The model under review builds one solid part; all positions refer to its coordinate system, in mm. Face numbers are marked on the shaded views. Coordinates: 2 decimals unless noted, no trailing zeros. Order: outer loops, then holes, each group sorted by start corner. A loop starts at its lowest first (then second) coordinate and runs counter-clockwise, first axis right, second up. Notation, with made-up numbers: (45, 20.5) -> (51, 20.5) arc R17 ccw to (51, 38.5) -> close; hole circle Ø8 at (-30.5, -14). An arc over 180 degrees is marked (long way). Answer as CSV lines item,"result". Start each with the question number.
from build123d import *

# Parameters (mm, degrees)
SKETCH1_R           = 52.832
SKETCH1_R_2         = 50.8
BOSS_EXTRUDE1_DEPTH = 457.2
CUT_EXTRUDE1_DEPTH  = 464.264805967
CIRPATTERN1_COUNT   = 8


with BuildPart() as part:
    # Sketch1 → Boss-Extrude1 (new body)
    with BuildSketch(Plane(origin=(0, 0, 0), x_dir=(1, 0, 0), z_dir=(0, 1, 0))):
        with Locations(Location((0, 0, 0), (0, 0, 270))):
            Circle(SKETCH1_R)
        with Locations(Location((0, 0, 0), (0, 0, 270))):
            Circle(SKETCH1_R_2, mode=Mode.SUBTRACT)
    extrude(amount=BOSS_EXTRUDE1_DEPTH)

    # Sketch2 → Cut-Extrude1 (cut, through all)
    with BuildSketch(Plane.XY):
        with BuildLine():
            Line((-9.525, 149.225), (-9.525, 0))
            Line((-9.525, 0), (9.525, 0))
            Line((9.525, 0), (9.525, 149.225))
            ThreePointArc((9.525, 149.225), (0, 158.75), (-9.525, 149.225))
        make_face()
    extrude(amount=CUT_EXTRUDE1_DEPTH, mode=Mode.SUBTRACT)

    # Sketch4 → 1/4 Clearance Hole1 (revolve, cut)
    with BuildSketch(Plane(origin=(0, 38.1, -52.832), x_dir=(0, 1, 0), z_dir=(1, 0, 0))):
        Polygon((0, 0), (0, 12.813817477), (3.57124, 10.668), (3.57124, 0), align=None)
    f_1_4_clearance_hole1 = revolve(axis=Axis((0, 38.1, -59.182), (0, 0, 1)), mode=Mode.SUBTRACT)

    # CirPattern1: 1/4 Clearance Hole1 ×8 about axis, 1 skipped
    cirpattern1_axis = Axis((0, 457.2, 0), (0, -1, 0))
    add([f_1_4_clearance_hole1.rotate(cirpattern1_axis, i * 360 / CIRPATTERN1_COUNT) for i in range(1, CIRPATTERN1_COUNT) if i not in (4,)], mode=Mode.SUBTRACT)


solid = part.part
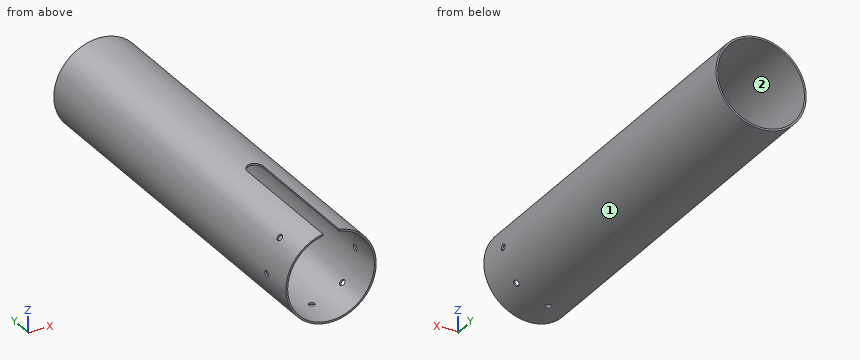
1) Consider section A-A (z = -17.5). Give the boundary of the cut face in (x, y).
2) Insertion check: pin 1 Ø6 at (y, z) = (318.5, -33.5) entering from +X; pin 2 Ø10 at (x, y) = (-41.5, 97.5) entering from +Z; pin 3 Ø4 at (y, z) = (383.5, 41) entering from -X. Each pin has a flat end and moves straight along its axis. Give the tip position at first contact, or say it passes through.
3) Consider section D-D (y = 122). Give the boundary of the cut face in (x, z) (3 decimals).
4) Consider section C-C (x = -26). Give the boundary of the cut face in (y, z), plus the area to 3 significant figures.
5) Wall thickness on L1, parallel to X at y = 365, z = 0; L2, parallel to Z at x = -3, y = 339.5; L3, parallel to X at y = 119, z = 34: over which ranges is each line inside the solid? List them lowest first. Write a range as [from, to].
6) Mouldability with a two-part tool opening along X and no side actions: class the marked faces 1 and 2 as released by +X, released by -X, zero draft, split by the parting line, or undercut.
7) Consider section B-B (y = 311). Give the boundary of the cut face in (x, z), plus the area to 3 significant figures.
Result:
1,outline,"(-49.85, 0) -> (-47.69, 0) -> (-47.69, 457.2) -> (-49.85, 457.2) -> close; (47.69, 0) -> (49.85, 0) -> (49.85, 457.2) -> (47.69, 457.2) -> close"
2,pin 1,"x = 43.14"
2,pin 2,"z = 38.2"
2,pin 3,"x = -35.64"
3,outline,"(-9.525, 49.899) -> (-9.525, 51.966) arc R52.832 ccw (long way) to (9.525, 51.966) -> (9.525, 49.899) arc R50.8 cw (long way) to start"
4,outline,"(0, -45.99) -> (457.2, -45.99) -> (457.2, -43.64) -> (0, -43.64) -> close; (0, 43.64) -> (457.2, 43.64) -> (457.2, 45.99) -> (0, 45.99) -> close"
4,area,"2,150 mm2"
5,L1,"[-52.83, -50.8], [50.8, 52.83]"
5,L2,"[-52.75, -50.71], [50.71, 52.75]"
5,L3,"[-40.44, -37.74], [37.74, 40.44]"
6,face 1,"split by the parting line"
6,face 2,"undercut"
7,outline,"circle Ø105.66 at (0, 0); hole circle Ø101.6 at (0, 0)"
7,area,"662 mm2"
